For this review, use the dimensioned drawing (mm, ordinates from the lowest corner) and the shaded views. A direction names the side the tool comes from. Coordinates: 2 decimals unless noted, no trailing zeros. Loops run counter-clockwise (first coordinate to the right, second up) from the corner with the lowest first, then second, coordinate; pieces in that order, holes last. Notation, with made-up numbers: (74.25, -38.5) - (118.25, -38.5) arc R24 ccw to (118.25, -24.5) - close; hole circle Ø1 at (65, 8). An arc over 180 degrees is marked (long way). Answer in a Markdown table with one row per item. Add a question column.
(1) For line 1 along Z through (x, y) = (1.2, 4); line 2 along Y through (x, z) = (0.4, 0.5), list the stretches that pass through material, from the lowest coordinate up.
(2) Mouldability with a two-part tool opening along X and no side actions: class the marked faces 3, 4, 5 and 6 as +X half, -X half, draft (parallel to the pull), parting line (faces both ways), or undercut.
(3) We need section C-C on z = 1.65. Write out the cut boundary in (x, y).
(4) We need section A-A on x = 1.9. Write out the cut boundary in (y, z), plus the area to 3 significant figures.
(5) We need section B-B on y = 5.75. Write out the cut boundary in (x, z), plus the area to 3 significant figures.
(6) Machinability: for the marked faces 1 and 2, which of the approach directions +Z, -Z, +X, -X, +Y, -Y give a long, thin tool a straight path to every point of the face, cutting with its end or side? Answer none if there is none.
(7) We need section D-D on z = 0.45. Write out the cut boundary in (x, y), plus the area to 3 significant figures.
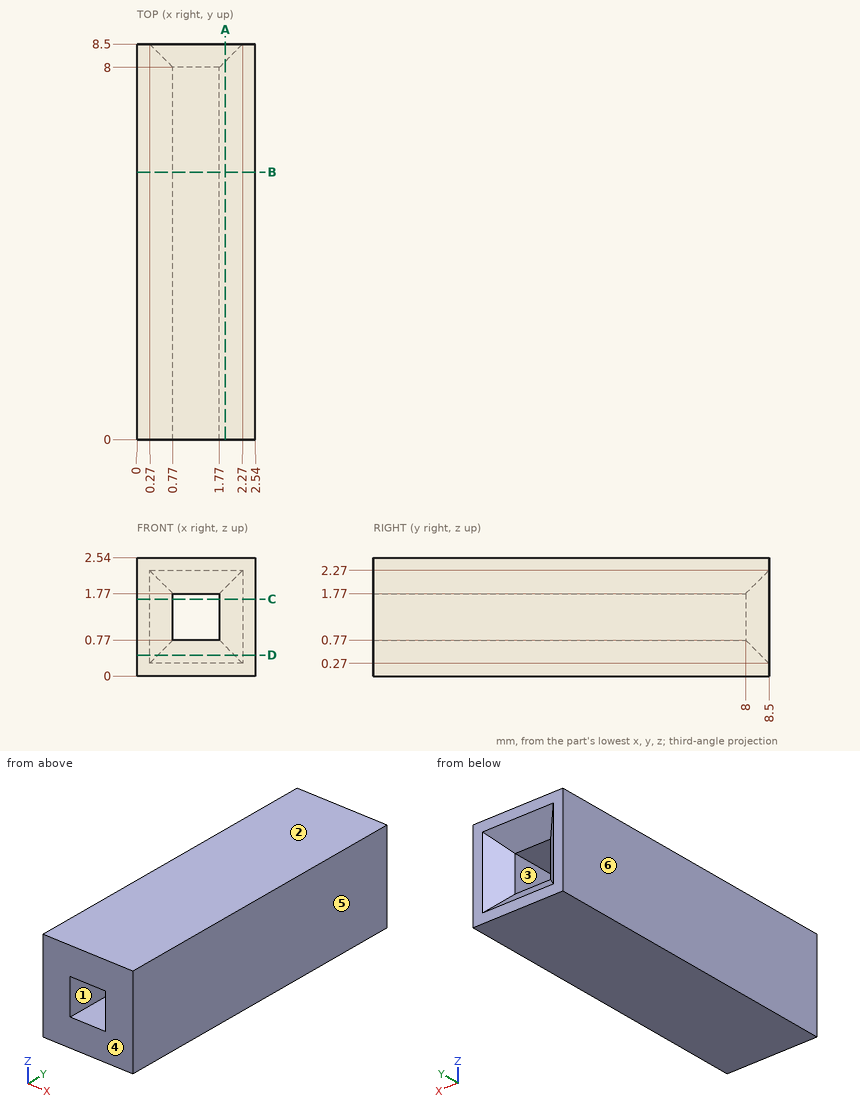
Outcome:
| question | item | result |
|---|---|---|
| 1 | line 1 | 0 to 0.77, 1.77 to 2.54 |
| 1 | line 2 | 0 to 8.37 |
| 2 | face 3 | undercut |
| 2 | face 4 | draft |
| 2 | face 5 | +X half |
| 2 | face 6 | -X half |
| 3 | outline | (0, 0) - (0.77, 0) - (0.77, 8) - (0.27, 8.5) - (0, 8.5) - close; (1.77, 0) - (2.54, 0) - (2.54, 8.5) - (2.27, 8.5) - (1.77, 8) - close |
| 4 | outline | (0, 0) - (8.5, 0) - (8.5, 0.27) - (8.13, 0.64) - (8.13, 1.9) - (8.5, 2.27) - (8.5, 2.54) - (0, 2.54) - close |
| 4 | area | 21.0 mm² |
| 5 | outline | (0, 0) - (2.54, 0) - (2.54, 2.54) - (0, 2.54) - close; hole (0.77, 0.77) - (1.77, 0.77) - (1.77, 1.77) - (0.77, 1.77) - close |
| 5 | area | 5.45 mm² |
| 6 | face 1 | +Y, -Y |
| 6 | face 2 | +Z, +X, -X, +Y, -Y |
| 7 | outline | (0, 0) - (2.54, 0) - (2.54, 8.5) - (2.27, 8.5) - (2.09, 8.32) - (0.45, 8.32) - (0.27, 8.5) - (0, 8.5) - close |
| 7 | area | 21.3 mm² |
